Work out the finished part from the listing and answer in its coordinate system (mm). A direction names the side the tool comes from. Coordinates: 2 decimals unless noted, no trailing zeros. Write each loop counter-clockwise with the first axis right and the second up, starting at its lowest first coordinate (ties: lowest second). Pieces come first, ordered by that corner, then holes. Notation, with made-up numbers: (49.5, 23.5) - (61.5, 23.5) arc R21 cw to (61.5, 28.5) - close; hole circle Ø1 at (-15.5, -34). An arc over 180 degrees is marked (long way). One line per item, written item: value.
Autodesk Inventor part; units mm, degrees
ref_plane "YZ Plane" through (0, 0, 0) normal (1, 0, 0) x (0, 1, 0)
ref_plane "XZ Plane" through (0, 0, 0) normal (0, 1, 0) x (-1, 0, 0)
ref_plane "XY Plane" through (0, 0, 0) normal (0, 0, 1) x (1, 0, 0)
sketch "Эскиз1" plane through (0, 0, 0) normal (0, 1, 0) x (-1, 0, 0)
  arc A0 (41, -50) -> (45.5, -45.5) centre (41, -45.5) ccw
  line L0 (0, -50) -> (41, -50)
  arc A1 (-4.5, -45.5) -> (0, -50) centre (0, -45.5) ccw
  line L1 (-4.5, -4.5) -> (-4.5, -45.5)
  arc A2 (0, 0) -> (-4.5, -4.5) centre (0, -4.5) ccw
  line L2 (-1.5, -45.5) -> (-1.5, -4.5)
  arc A3 (0, -3) -> (-1.5, -4.5) centre (0, -4.5) ccw
  line L3 (0, -3) -> (41, -3)
  line L4 (41, 0) -> (0, 0)
  arc A4 (45.5, -4.5) -> (41, 0) centre (41, -4.5) ccw
  line L5 (45.5, -45.5) -> (45.5, -4.5)
  line L6 (42.5, -4.5) -> (42.5, -45.5)
  arc A5 (42.5, -4.5) -> (41, -3) centre (41, -4.5) ccw
  line L7 (41, -47) -> (0, -47)
  arc A6 (41, -47) -> (42.5, -45.5) centre (41, -45.5) ccw
  arc A7 (-1.5, -45.5) -> (0, -47) centre (0, -45.5) ccw
  circle A8 centre (20.5, -25) radius 18.5
  circle A9 centre (20.5, -25) radius 16.5
  circle A10 centre (20.5, -25) radius 14.5
  circle A11 centre (20.5, -25) radius 13.5
  point P0 (11.5, -30)
extrude "Выдавливание1" add sketch "Эскиз1" along normal blind 10 contours L2 A3 L3 A5 L6 A6 L7 A7 | A8 | A9 | A10 | A11
extrude "Выдавливание2" cut sketch "Эскиз1" along normal blind 3 contours A8 | A10
properties part number "Cap" material "Стекло, литое, серое"
Item 1: Consider probe 1 along Z at (x, y) = (-20.5, 2.35); probe 2 along Y at (x, z) = (-32.5, -12); probe 3 along X at (y, z) = (1.75, -29). Determine where each line is inside the solid, lowest interval first.
Evaluation:
probe 1: z = -47 to -43.5, -41.5 to -39.5, -38.5 to -11.5, -10.5 to -8.5, -6.5 to -3
probe 2: y = 3 to 10
probe 3: x = -42.5 to -38.56, -36.51 to -34.44, -33.39 to -7.61, -6.56 to -4.49, -2.44 to 1.5
Item 2: Section D-D, the plane x = -5 is taken. Determine the outline of the cut face in (y, z), then the cut area to 3 significant figures.
Evaluation:
outline: (0, -47) - (10, -47) - (10, -3) - (0, -3) - (0, -14.9) - (3, -14.9) - (3, -19.34) - (0, -19.34) - (0, -30.66) - (3, -30.66) - (3, -35.1) - (0, -35.1) - close
area: 413 mm2
Item 3: Section B-B, the plane x = -20.5 is taken. Determine the outline of the cut face in (y, z).
Evaluation:
outline: (0, -47) - (10, -47) - (10, -3) - (0, -3) - (0, -6.5) - (3, -6.5) - (3, -8.5) - (0, -8.5) - (0, -10.5) - (3, -10.5) - (3, -11.5) - (0, -11.5) - (0, -38.5) - (3, -38.5) - (3, -39.5) - (0, -39.5) - (0, -41.5) - (3, -41.5) - (3, -43.5) - (0, -43.5) - close
Item 4: Section C-C, the plane z = -25 is taken. Determine the outline of the cut face in (x, y), then the cut area to 3 significant figures.
Evaluation:
outline: (-42.5, 0) - (-39, 0) - (-39, 3) - (-37, 3) - (-37, 0) - (-35, 0) - (-35, 3) - (-34, 3) - (-34, 0) - (-7, 0) - (-7, 3) - (-6, 3) - (-6, 0) - (-4, 0) - (-4, 3) - (-2, 3) - (-2, 0) - (1.5, 0) - (1.5, 10) - (-42.5, 10) - close
area: 422 mm2
Item 5: Section A-A, the plane z = -7.5 is taken. Determine the outline of the cut face in (x, y).
Evaluation:
outline: (-42.5, 0) - (-26.5, 0) - (-26.5, 3) - (-14.5, 3) - (-14.5, 0) - (1.5, 0) - (1.5, 10) - (-42.5, 10) - close
Item 6: Which of the six approach directions +Z, -Z, +X, -X, +Y, -Y give full straight-line access (tool end or side, diameter ignored) to faces 1 (the face through (-25, 3, -38)), 2 (the face through (1.07, 4.93, -3.45))?
Evaluation:
face 1: -Y
face 2: +Z, +X, +Y, -Y
